CAD build for the part. Positions are in the model's coordinates, mm. A direction names the side the tool comes from. Round coordinates to 2 decimals unless told otherwise and drop trailing zeros. Loops run counter-clockwise (first coordinate to the right, second up) from the corner with the lowest first, then second, coordinate; pieces in that order, holes last.
```python
from build123d import *

# Parameters (mm, degrees)
SKETCH1_W           = 30
SKETCH1_H           = 50
SKETCH1_W_2         = 22
SKETCH1_H_2         = 25
BOSS_EXTRUDE1_DEPTH = 1.45


with BuildPart() as part:
    # Sketch1 → Boss-Extrude1 (new, symmetric)
    with BuildSketch(Plane.XY):
        with Locations((15, 25)):
            Rectangle(SKETCH1_W, SKETCH1_H)
        with BuildLine():
            Line((4.6, 44), (7.6, 44))
            ThreePointArc((7.6, 44), (9.1, 42.5), (7.6, 41))
            Line((7.6, 41), (4.6, 41))
            ThreePointArc((4.6, 41), (3.1, 42.5), (4.6, 44))
        make_face(mode=Mode.SUBTRACT)
        with BuildLine():
            Line((25.4, 44), (22.4, 44))
            ThreePointArc((22.4, 44), (20.9, 42.5), (22.4, 41))
            Line((22.4, 41), (25.4, 41))
            ThreePointArc((25.4, 41), (26.9, 42.5), (25.4, 44))
        make_face(mode=Mode.SUBTRACT)
        with Locations((15, 22.5)):
            Rectangle(SKETCH1_W_2, SKETCH1_H_2, mode=Mode.SUBTRACT)
    extrude(amount=BOSS_EXTRUDE1_DEPTH, both=True)


solid = part.part
```
Item 1: Cut at A-A, the plane y = 15.5. Give the cut face in (x, z), plus the area to 3 significant figures.
Answers follow:
outline: (0, -1.45) - (4, -1.45) - (4, 1.45) - (0, 1.45) - close; (26, -1.45) - (30, -1.45) - (30, 1.45) - (26, 1.45) - close
area: 23.2 mm2
Item 2: Cut at B-B, the plane z = -0.45. Give the cut face in (x, y), plus the area to 3 significant figures.
Answers follow:
outline: (0, 0) - (30, 0) - (30, 50) - (0, 50) - close; hole (4, 10) - (26, 10) - (26, 35) - (4, 35) - close; hole (4.6, 41) - (7.6, 41) arc R1.5 ccw to (7.6, 44) - (4.6, 44) arc R1.5 ccw to start; hole (22.4, 41) - (25.4, 41) arc R1.5 ccw to (25.4, 44) - (22.4, 44) arc R1.5 ccw to start
area: 918 mm2
Item 3: Cut at C-C, the plane x = 23.75. Give the cut face in (y, z).
Answers follow:
outline: (0, -1.45) - (10, -1.45) - (10, 1.45) - (0, 1.45) - close; (35, -1.45) - (41, -1.45) - (41, 1.45) - (35, 1.45) - close; (44, -1.45) - (50, -1.45) - (50, 1.45) - (44, 1.45) - close
Item 4: Cut at D-D, the plane y = 42.5. Give the cut face in (x, z), plus the area to 3 significant figures.
Answers follow:
outline: (0, -1.45) - (3.1, -1.45) - (3.1, 1.45) - (0, 1.45) - close; (9.1, -1.45) - (20.9, -1.45) - (20.9, 1.45) - (9.1, 1.45) - close; (26.9, -1.45) - (30, -1.45) - (30, 1.45) - (26.9, 1.45) - close
area: 52.2 mm2
Item 5: 3-axis set-ups, long thin cutter, end or side, ignore diameter. For faces 4 (the flat face through (15, 36, 1.45)), 5 (the flat face through (6, 41, 0)): which of +Z, -Z, +X, -X, +Y, -Y reach the whole face in a straight line?
Answers follow:
face 4: +Z, +X, -X, +Y, -Y
face 5: +Z, -Z
Item 6: Probe line 1 (X direction, y = 16.5, z = 0.35); line 2 (Y direction, x = 16.25, z = 0); line 3 (Y direction, x = 21.5, z = 0.25). List the from-to ranges inside material, lowest first.
Answers follow:
line 1: x = 0 to 4, 26 to 30
line 2: y = 0 to 10, 35 to 50
line 3: y = 0 to 10, 35 to 41.3, 43.7 to 50
Item 7: Two-plate mould, pull along Y, no slides. Class faces 1 (the flat face through (15, 36, -1.45)), 2 (the flat face through (15, 50, 0)), 3 (the flat face through (6, 44, 0)): released by +Y, released by -Y, zero draft, split by the parting line, or undercut.
Answers follow:
face 1: zero draft
face 2: released by +Y
face 3: undercut
